from build123d import *

# Parameters (mm, degrees)
EXTRUDE1_DEPTH     = 21.59
EXTRUDE2_DEPTH     = 16.51
SKETCH4_W          = 146.050000002
SKETCH4_H          = 21.59
CUT_EXTRUDE2_DEPTH = 5.08
SKETCH6_R          = 3.302000001
SKETCH6_R_2        = 3.302
CUT_EXTRUDE3_DEPTH = 5.08
SKETCH3_R          = 1.5875
CUT_EXTRUDE1_DEPTH = 21.59


with BuildPart() as part:
    # Sketch2 → Extrude1 (new body)
    with BuildSketch(Plane.XY):
        Polygon((839.47, -5504.129603175), (839.47, -5314.95), (174.9425, -5314.95), (174.9425, -5573.445396825), align=None)
    extrude(amount=-EXTRUDE1_DEPTH)

    # Sketch7 → Extrude2 (add)
    with BuildSketch(Plane(origin=(0, 0, -21.59), x_dir=(-1, 0, 0), z_dir=(0, 0, -1))):
        Polygon((-174.9425, -5314.95), (-153.3525, -5314.95), (-153.3525, -5575.697414966), (-174.9425, -5573.445396825), align=None)
        Polygon((-839.47, -5314.95), (-861.06, -5314.95), (-861.06, -5501.877585034), (-839.47, -5504.129603175), align=None)
    extrude(amount=-EXTRUDE2_DEPTH)

    # Sketch4 → Cut-Extrude2 (cut)
    with BuildSketch(Plane.XY):
        with Locations((522.2875, -5415.661000001)):
            Rectangle(SKETCH4_W, SKETCH4_H)
    extrude(amount=-CUT_EXTRUDE2_DEPTH, mode=Mode.SUBTRACT)

    # Sketch6 → Cut-Extrude3 (cut)
    with BuildSketch(Plane.XY):
        with Locations((451.507564029, -5407.111064031)):
            Circle(SKETCH6_R)
        with Locations((451.507564029, -5424.210935971)):
            Circle(SKETCH6_R_2)
        with Locations((593.067435971, -5424.210935971)):
            Circle(SKETCH6_R_2)
        with Locations((593.067435971, -5407.111064031)):
            Circle(SKETCH6_R)
    extrude(amount=-CUT_EXTRUDE3_DEPTH, mode=Mode.SUBTRACT)

    # Sketch3 → Cut-Extrude1 (cut)
    with BuildSketch(Plane.XY):
        with Locations((166.0525, -5531.135582009)):
            Circle(SKETCH3_R)
        with Locations((166.0525, -5444.661349205)):
            Circle(SKETCH3_R)
        with Locations((166.0525, -5358.187116401)):
            Circle(SKETCH3_R)
        with Locations((848.36, -5471.826917991)):
            Circle(SKETCH3_R)
        with Locations((848.36, -5409.076150795)):
            Circle(SKETCH3_R)
        with Locations((848.36, -5346.325383599)):
            Circle(SKETCH3_R)
        with Locations((573.0875, -5417.566)):
            Circle(SKETCH3_R)
        with Locations((522.2875, -5417.566)):
            Circle(SKETCH3_R)
        with Locations((471.4875, -5417.566)):
            Circle(SKETCH3_R)
    extrude(amount=-CUT_EXTRUDE1_DEPTH, mode=Mode.SUBTRACT)


solid = part.part
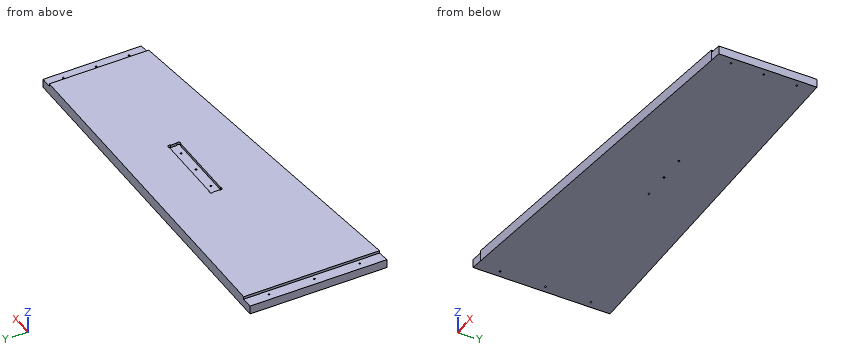
Could you check a few things on this model? Use its own coordinates, in mm. Give positions to 0.01 mm unless a question says otherwise; leave off trailing zeros. Write each loop counter-clockwise with the first axis right and the second up, starting at its lowest first coordinate (ties: lowest second). Pieces come first, ordered by that corner, then holes. Notation, with made-up numbers: (7.25, 40.5) - (49.25, 40.5) arc R22 ccw to (49.25, 56.5) - close; hole circle Ø6 at (-1.5, 6.5). An arc over 180 degrees is marked (long way). Use CSV: the item, a comma, the result in double quotes. Start each with the question number.
Item 1: I'm going to push flat-ended pins straight in: pin 1 (3 mm diameter, centred on x = 166.05, y = -5531.14, fed in from -Z); pin 2 (1 mm diameter, centred on x = 599, z = -18, fed in from -Y); pin 3 (5.5 mm diameter, centred on x = 500.5, z = -1.5, fed in from -Y); pin 4 (4 mm diameter, centred on x = 471.49, y = -5417.57, fed in from +Z). Where does each tip first touch, or does it pass through?
Item 2: I want a section at A-A, the plane z = -11. Give the number of separate pieces and of enclosed holes in the cut face, then the cut area to 3 significant figures.
Item 3: I want a section at B-B, the plane x = 422. Please give me the cut outline in (y, z).
Item 4: I want a section at C-C, the plane x = 805. Please give me the cut outline in (y, z).
Item 5: If I drill on line 1 along Y through (x, z) = (848.36, -9.25); line 2 along X through (y, z) = (-5346.5, -11); line 3 along Y through (x, z) = (547, -3.75), over which ranges is the centre line in solid material (lowest first)?
Findings:
1,pin 1,"passes through"
1,pin 2,"stops at y = -5529.26"
1,pin 3,"stops at y = -5539.77"
1,pin 4,"stops at z = -5.08"
2,separate pieces,"1"
2,enclosed holes,"9"
2,area,"158,000 mm2"
3,outline,"(-5547.68, -21.59) - (-5314.95, -21.59) - (-5314.95, 0) - (-5547.68, 0) - close"
4,outline,"(-5507.73, -21.59) - (-5314.95, -21.59) - (-5314.95, 0) - (-5507.73, 0) - close"
5,line 1,"y = -5503.2 to -5473.41, -5470.24 to -5410.66, -5407.49 to -5347.91, -5344.74 to -5314.95"
5,line 2,"x = 153.35 to 846.78, 849.94 to 861.06"
5,line 3,"y = -5534.64 to -5426.46, -5404.87 to -5314.95"
